Geometry check sheet. Reference: the model listing, model coordinates, mm. A direction names the side the tool comes from. Give positions to 0.01 mm unless a question says otherwise; leave off trailing zeros. Order: outer loops, then holes, each group sorted by start corner. A loop starts at its lowest first (then second) coordinate and runs counter-clockwise, first axis right, second up. Notation, with made-up numbers: M -10,-37 L 12,-37 A26 ccw 12,-18 Z; hole C -28,-27 d1. An arc over 180 degrees is marked long. Put each result on its own line as item: value. Start each with the question number.
Q1. Section check C-C on z = 30.5. Record the cut outline in (x, y) (3 decimals).
Q2. Mould release check, pull along X, two halves, no side actions. Record for faces 3 (the flat face through (0, 22.225, 1)), 4 (the flat face through (-12.7, 0, 1)), 5 (the flat face through (-10, -2, -76.2)): +X half, -X half, draft (parallel to the pull), parting line (faces both ways), or undercut.
Q3. Section check A-A on x = 7.5. Record the cut outline in (y, z) (3 decimals), then the cut area to 3 significant figures.
Q4. Material ranges on L1, parallel to X at y = -20, z = 56 (3 decimals); L2, parallel to Y at x = -2.5, z = -26 (3 decimals), recorded low to high.
Q5. Section check B-B on y = 4.5. Record the cut outline in (x, z) (3 decimals).
Q6. Access from +Z, -Z, +X, -X, +Y, -Y to the whole of each face (thin tool, end or side, straight path). Record for faces 1 (the flat face through (-9.525, 0, 1)), 2 (the cylindrical face through (-11.135, 10.208, 21.745)).
Q7. Go/stop test with a flat-tipped pin: pin 1 (4 mm diameter, centred on y = -12.7, z = 22.3, fed in from +X). Record where the tip stops, or that it passes through.
Q8. Section check D-D on y = -12.7. Record the cut outline in (x, z) (3 decimals), then the cut area to 3 significant figures.
```python
from build123d import *

# Parameters (mm, degrees)
SKETCH1_W              = 25.4
SKETCH1_H              = 50.8
SKETCH1_W_2            = 19.05
SKETCH1_H_2            = 44.45
BOSS_EXTRUDE1_DEPTH    = 76.2
F_10_CLEARANCE_HOLE1_D = 5.1054


with BuildPart() as part:
    # Sketch1 → Boss-Extrude1 (new, symmetric)
    with BuildSketch(Plane.XY):
        Rectangle(SKETCH1_W, SKETCH1_H)
        Rectangle(SKETCH1_W_2, SKETCH1_H_2, mode=Mode.SUBTRACT)
    extrude(amount=BOSS_EXTRUDE1_DEPTH, both=True)

    # #10 Clearance Hole1 (through all)
    with Locations(Plane(origin=(12.7, 0, 0), x_dir=(0, 0, -1), z_dir=(1, 0, 0))):
        with Locations((-22.298769885, 12.7), (28.501230115, 12.7), (28.501230115, -12.7), (-22.298769885, -12.7)):
            Hole(F_10_CLEARANCE_HOLE1_D / 2)


solid = part.part
```
Results found:
1. outline: M -12.7,-25.4 L 12.7,-25.4 L 12.7,25.4 L -12.7,25.4 Z; hole M -9.525,-22.225 L 9.525,-22.225 L 9.525,22.225 L -9.525,22.225 Z
2. face 3: undercut
2. face 4: -X half
2. face 5: draft
3. outline: M -25.4,-76.2 L -22.225,-76.2 L -22.225,76.2 L -25.4,76.2 Z; M 22.225,-76.2 L 25.4,-76.2 L 25.4,76.2 L 22.225,76.2 Z
3. area: 968 mm^2
4. L1: x = -12.7 to -9.525, 9.525 to 12.7
4. L2: y = -25.4 to -22.225, 22.225 to 25.4
5. outline: M -12.7,-76.2 L -9.525,-76.2 L -9.525,76.2 L -12.7,76.2 Z; M 9.525,-76.2 L 12.7,-76.2 L 12.7,76.2 L 9.525,76.2 Z
6. face 1: +Z, -Z
6. face 2: +X, -X
7. pin 1: passes through
8. outline: M -12.7,-76.2 L -9.525,-76.2 L -9.525,-31.054 L -12.7,-31.054 Z; M -12.7,-25.949 L -9.525,-25.949 L -9.525,19.746 L -12.7,19.746 Z; M -12.7,24.851 L -9.525,24.851 L -9.525,76.2 L -12.7,76.2 Z; M 9.525,-76.2 L 12.7,-76.2 L 12.7,-31.054 L 9.525,-31.054 Z; M 9.525,-25.949 L 12.7,-25.949 L 12.7,19.746 L 9.525,19.746 Z; M 9.525,24.851 L 12.7,24.851 L 12.7,76.2 L 9.525,76.2 Z
8. area: 903 mm^2
